from build123d import *

# Parameters (mm, degrees)
SKETCH2_R           = 2.3
SKETCH2_R_2         = 1.1
BOSS_EXTRUDE1_DEPTH = 7


with BuildPart() as part:
    # Sketch2 → Boss-Extrude1 (new body)
    with BuildSketch(Plane.XY):
        with BuildLine():
            Line((16.77037128, 5), (46.77037128, 5))
            ThreePointArc((46.77037128, 5), (51.770370099, 0), (46.77037128, -5))
            Line((46.77037128, -5), (24.516048425, -5))
            ThreePointArc((24.516048425, -5), (24.330990192, -5.124148498), (24.375678975, -5.342465496))
            Line((24.375678975, -5.342465496), (26.419446474, -7.35616374))
            ThreePointArc((26.419446474, -7.35616374), (26.580741343, -7.462645583), (26.770370099, -7.5))
            Line((26.770370099, -7.5), (46.77037187, -7.5))
            ThreePointArc((46.77037187, -7.5), (54.270370099, 2.95e-07), (46.77037128, 7.5))
            Line((46.77037128, 7.5), (-0.729629901, 7.5))
            ThreePointArc((-0.729629901, 7.5), (-8.229629901, 0), (-0.729629901, -7.5))
            Line((-0.729629901, -7.5), (16.770370099, -7.5))
            ThreePointArc((16.770370099, -7.5), (16.95577733, -7.374994391), (16.909415122, -7.156241586))
            Line((16.909415122, -7.156241586), (13.261135036, -3.561637402))
            ThreePointArc((13.261135036, -3.561637402), (12.143915454, 1.896287556), (16.77037128, 5))
        make_face()
        with Locations((1.770370689, 0)):
            Circle(SKETCH2_R, mode=Mode.SUBTRACT)
        with Locations((8.620370689, 0)):
            Circle(SKETCH2_R_2, mode=Mode.SUBTRACT)
        with Locations((-5.079629311, 0)):
            Circle(SKETCH2_R_2, mode=Mode.SUBTRACT)
    extrude(amount=BOSS_EXTRUDE1_DEPTH)


solid = part.part
Geometry: final body of the model. Coordinates: model frame, mm. A direction names the side the tool comes from. Round coordinates to 2 decimals unless told otherwise and drop trailing zeros. Loops run counter-clockwise (first coordinate to the right, second up) from the corner with the lowest first, then second, coordinate; pieces in that order, holes last. Notation, with made-up numbers: M 48.25,13 L 65.25,13 A18 cw 65.25,30 Z; hole C 26.25,85 d9. An arc over 180 degrees is marked long. One line per question, with ' | ' between items.
(1) Contact query for flat-ended pins moving along their axis: P1, Ø3, axis at x = 41, y = 4.5, coming from the +Z side; P2, Ø2, axis at x = 24.5, z = 4, coming from the -Y side; P3, Ø1, axis at y = 5, z = 5.5, coming from the +X side. Output: stop coordinate, or through.
Check result:
P1: stops at z = 7 | P2: stops at y = -6.45 | P3: stops at x = 52.77
(2) Material intervals for line 1 along X through (y, z) = (1, 1.75); line 2 along Y through (x, z) = (40, 1.5); line 3 along X through (y, z) = (1.5, 0.5), sorted ascending. Write a range as from..to.
Check result:
line 1: x = -8.16..-5.54, -4.62..-0.3, 3.84..8.16, 9.08..11.87, 51.67..54.2 | line 2: y = -7.5..-5, 5..7.5 | line 3: x = -8.08..0.03, 3.51..12, 51.54..54.12
(3) Cut plane A-A on y = 0. Return the cut outline in (x, z), plus the area to 3 significant figures.
Check result:
outline: M -8.23,0 L -6.18,0 L -6.18,7 L -8.23,7 Z; M -3.98,0 L -0.53,0 L -0.53,7 L -3.98,7 Z; M 4.07,0 L 7.52,0 L 7.52,7 L 4.07,7 Z; M 9.72,0 L 11.77,0 L 11.77,7 L 9.72,7 Z; M 51.77,0 L 54.27,0 L 54.27,7 L 51.77,7 Z | area: 94.5 mm2
(4) Pull-direction query (X, two-part tool) for faces 1 (the cylindrical face through (-8.228, 0.165, 3.451)), 2 (the flat face through (36, -5, 3)), 3 (the flat face through (15.6, 5.1, 0)); classes: +X half, -X half, draft (parallel to the pull), parting line (faces both ways), or undercut.
Check result:
face 1: -X half | face 2: undercut | face 3: draft
(5) Access query for faces 4 (the cylindrical face through (12.113, 1.819, 3.451)), 5 (the flat face through (25.383, -6.335, 3.451)), 6 (the flat face through (8, -7.5, 3)). Directions: +Z, -Z, +X, -X, +Y, -Y. A direction counts if a zero-diameter tool reaches every point of the face in a straight line with its end or side. Return the directions, or none.
Check result:
face 4: +Z, -Z | face 5: +Z, -Z, -Y | face 6: +Z, -Z, +X, -X, -Y
(6) Cut plane C-C on z = 1.5. Return the cut outline in (x, y), plus the area to 3 significant figures.
Check result:
outline: M -0.73,-7.5 L 16.77,-7.5 A0.2 ccw 16.91,-7.16 L 13.26,-3.56 A5 cw 16.77,5 L 46.77,5 A5 cw 46.77,-5 L 24.52,-5 A0.2 ccw 24.38,-5.34 L 26.42,-7.36 A0.5 ccw 26.77,-7.5 L 46.77,-7.5 A7.5 ccw 46.77,7.5 L -0.73,7.5 A7.5 ccw Z; hole C -5.08,0 d2.2; hole C 1.77,0 d4.6; hole C 8.62,0 d2.2 | area: 463 mm2
(7) Cut plane D-D on x = 15. Return the cut outline in (y, z).
Check result:
outline: M -7.5,0 L -5.27,0 L -5.27,7 L -7.5,7 Z; M 4.68,0 L 7.5,0 L 7.5,7 L 4.68,7 Z
(8) Cut plane B-B on x = 35.5. Return the cut outline in (y, z), plus the area to 3 significant figures.
Check result:
outline: M -7.5,0 L -5,0 L -5,7 L -7.5,7 Z; M 5,0 L 7.5,0 L 7.5,7 L 5,7 Z | area: 35.0 mm2
